from build123d import *
from build123d.topology import SkipClean

# Parameters (mm, degrees)
SKETCH_1_R          = 1.95
EXTRUDE_1_DEPTH     = 12
SKETCH_4_W          = 2
SKETCH_4_H          = 9
EXTRUDE_2_DEPTH     = 1.95
EXTRUDE_4_DEPTH     = 8.8
SKETCH_9_R          = 2
CUT_EXTRUDE_2_DEPTH = 17
SKETCH_13_R         = 2.75
CUT_EXTRUDE_6_DEPTH = 1
CUT_EXTRUDE_7_DEPTH = 13.389713
SKETCH_14_R         = 0.25
CUT_EXTRUDE_8_DEPTH = 15.053647


with BuildPart() as part:
    # 스케치1 → 보스-돌출1 (new body)
    with BuildSketch(Plane.XY):
        Circle(SKETCH_1_R)
    extrude(amount=EXTRUDE_1_DEPTH)

    # 스케치4 → 보스-돌출2 (add)
    with BuildSketch(Plane(origin=(0, 0, 0), x_dir=(0, 0, -1), z_dir=(1, 0, 0))):
        with Locations((-1, -2.55)):
            Rectangle(SKETCH_4_W, SKETCH_4_H)
    extrude(amount=EXTRUDE_2_DEPTH)

    # 스케치8 → 보스-돌출4 (add)
    with BuildSketch(Plane.XY.offset(2)):
        with BuildLine():
            ThreePointArc((1.95, -1.643168), (1.075273, -2.312204), (0, -2.55))
            Line((0, -2.55), (0, -7.05))
            Line((0, -7.05), (1.95, -7.05))
            Line((1.95, -7.05), (1.95, -1.643168))
        make_face()
    extrude(amount=EXTRUDE_4_DEPTH)

    # 스케치9 → 컷-돌출2 (cut)
    with BuildSketch(Plane.ZY):
        with Locations((5.5, -7.55)):
            Circle(SKETCH_9_R)
    extrude(amount=-CUT_EXTRUDE_2_DEPTH, mode=Mode.SUBTRACT)

    # 스케치13 → 컷-돌출6 (cut)
    with BuildSketch(Plane.ZY):
        with Locations((5.505014, -7.55)):
            Circle(SKETCH_13_R)
    extrude(amount=-CUT_EXTRUDE_6_DEPTH, mode=Mode.SUBTRACT)

    # 스케치12 → 컷-돌출7 (cut, through all)
    with BuildSketch(Plane.XY.offset(2)):
        with BuildLine():
            Line((1.95, 0), (1.95, 1.95))
            Line((1.95, 1.95), (0, 1.95))
            ThreePointArc((0, 1.95), (1.378858, 1.378858), (1.95, 0))
        make_face()
    extrude(amount=-CUT_EXTRUDE_7_DEPTH, mode=Mode.SUBTRACT)

    # 스케치14 → 컷-돌출8 (cut, through all)
    with SkipClean():  # the faces are left unmerged after this step: merging them gives an invalid solid
        with BuildSketch(Plane(origin=(0, 0, 0), x_dir=(-1, 0, 0), z_dir=(0, 0, -1))):
            with Locations((-0.975, -3.55)):
                Circle(SKETCH_14_R)
        extrude(amount=-CUT_EXTRUDE_8_DEPTH, mode=Mode.SUBTRACT)


solid = part.part
Design review of the part built by this model. Coordinates are the model's own, in mm. A direction names the side the tool comes from. Round coordinates to 2 decimals unless told otherwise and drop trailing zeros. Order: outer loops, then holes, each group sorted by start corner. A loop starts at its lowest first (then second) coordinate and runs counter-clockwise, first axis right, second up. Notation, with made-up numbers: M 88,-32.75 L 132,-32.75 A22 cw 132,-1.75 Z; hole C -4,-38 d6. An arc over 180 degrees is marked long. Answer as CSV lines item,"result". Start each with the question number.
1) The part is to be moulded in two halves that separate along Y. For faces 4 (the face through (1, -2, 2)), 5 (the face through (1, -7.05, 9)), 6 (the face through (0, -4, 5)), say which applies: +Y half, -Y half, draft (parallel to the pull), parting line (faces both ways), or undercut.
2) Add section B-B (z = 9). Give the boundary of the cut face in (x, y) (3 decimals), then the cut area to 3 significant figures.
3) For pin 1 Ø1 at (x, y) = (1, -5) entering from +Z; pin 2 Ø1.1 at (y, z) = (-5.5, 5.5) entering from -X; pin 3 Ø4 at (y, z) = (-3.5, 3) entering from -X, all flat-tipped, find the tip position at first contact; note any pin that passes through.
4) Tool access review of faces 1 (the face through (1.1, -2.3, 6.3)), 2 (the face through (1, -7.05, 2)), 3 (the face through (0.5, -4.8, 5.6)): name each direction out of +Z, -Z, +X, -X, +Y, -Y from which nothing blocks a thin tool from reaching the whole face with its end or side.
5) Add section C-C (y = -4.5). Give the boundary of the cut face in (x, z), then the cut area to 3 significant figures.
6) Add section D-D (z = 7). Give the boundary of the cut face in (x, y) (3 decimals).
7) Add section A-A (y = -3.55). Give the boundary of the cut face in (x, z) (3 decimals).
8) Wall thickness on line 1 along X through (y, z) = (-5.75, 6.75); line 2 along X through (y, z) = (-6, 10); line 3 along Y through (x, z) = (1.05, 5.25): over which ranges is each line inside the solid? List them lowest first. Write a range as [from, to].
Resolved:
1,face 4,"undercut"
1,face 5,"-Y half"
1,face 6,"draft"
2,outline,"C 0,0 d3.9; M 0,-7.05 L 1.95,-7.05 L 1.95,-1.643 A2.55 cw 0,-2.55 Z; hole C 0.975,-3.55 d0.5"
2,area,"21.1 mm^2"
3,pin 1,"z = 10.8"
3,pin 2,"x = 1"
3,pin 3,"x = -1.25"
4,face 1,"+Z"
4,face 2,"+Z, -Z, +X, -X, -Y"
4,face 3,"-X, -Y"
5,outline,"M 0,0 L 1.95,0 L 1.95,10.8 L 0,10.8 Z"
5,area,"21.1 mm^2"
6,outline,"C 0,0 d3.9; M 0,-5.242 L 1,-5.242 L 1,-6.227 L 1.95,-6.227 L 1.95,-1.643 A2.55 cw 0,-2.55 Z; hole C 0.975,-3.55 d0.5"
7,outline,"M 0,0 L 0.725,0 L 0.725,10.8 L 0,10.8 Z; M 1.225,0 L 1.95,0 L 1.95,10.8 L 1.225,10.8 Z"
8,line 1,"[1, 1.95]"
8,line 2,"[0, 1.95]"
8,line 3,"[-5.57, -3.79], [-3.31, -2.32], [-1.64, 1.64]"
